Geometry: final body of the model. Coordinates: model frame, mm. A direction names the side the tool comes from. Coordinates: 2 decimals unless noted, no trailing zeros. Write each loop counter-clockwise with the first axis right and the second up, starting at its lowest first coordinate (ties: lowest second). Pieces come first, ordered by that corner, then holes. Notation, with made-up numbers: M 5,78.25 L 24,78.25 A27 cw 24,100.25 Z; hole C 19.5,25.25 d10. An arc over 180 degrees is marked long. Write item = value, one per line. Start each with the question number.
Item 1: Ray query, L1, parallel to Y at x = 10, z = -15.5; L2, parallel to Z at x = 24.75, y = -16.5; L3, parallel to Z at x = 15.5, y = -2. Return the intervals inside material, ascending. Write a range as [from, to].
Item 2: Section C-C on z = -13. Output: boundary loops of the cut face in (x, y), plus the area to 3 significant figures.
Item 3: Section A-A on x = 18.25. Output: boundary loops of the cut face in (y, z).
Item 4: First-contact query: pin 1 Ø10 at (x, y) = (11, -11.5) entering from +Z; pin 2 Ø5 at (x, y) = (13, 9.5) entering from +Z; pin 3 Ø4 at (x, y) = (16.5, 10.5) entering from +Z. Flat tips, straight axial feed; report the tip coordinate or a pass-through.
Item 5: Section B-B on y = 34. Output: boundary loops of the cut face in (x, z), plus the area to 3 significant figures.
Item 6: Reachability of faces 1 (the flat face through (13, -44.45, -20)), 2 (the flat face through (12.52, -41.77, -15.41)) from +Z, -Z, +X, -X, +Y, -Y: full face, straight path, thin tool, end or side. Return the list, or none.
from build123d import *

# Parameters (mm, degrees)
F1_DEPTH = 25.4
F2_R     = 5.08


with BuildPart() as f1:
    # F0 (on Right) → F1 (new body)
    with BuildSketch(Plane.YZ):
        Polygon((-44.45, -15.24), (-44.45, -25.4), (44.45, -25.4), (44.45, 22.65116), (24.805692, 13.670905), (-41.259935, -16.530525), (-42.299335, -14.256839), align=None)
    extrude(amount=F1_DEPTH)

    # F2
    f2_edges = [f1.edges().sort_by_distance(p)[0] for p in [
        (12.7, 44.45, 22.65116),
    ]]
    fillet(f2_edges, radius=F2_R)


solid = f1.part
Responses:
q1.L1 = [-44.45, -41.73], [-39.01, 44.45]
q1.L2 = [-25.4, -5.21]
q1.L3 = [-25.4, 1.42]
q2.outline = M 0,-33.54 L 25.4,-33.54 L 25.4,44.45 L 0,44.45 Z
q2.area = 1,980 mm²
q3.outline = M -44.45,-25.4 L 44.45,-25.4 L 44.45,14.74 A5.08 ccw 37.26,19.36 L -41.26,-16.53 L -42.3,-14.26 L -44.45,-15.24 Z
q4.pin_1 = -0.64
q4.pin_2 = 7.82
q4.pin_3 = 8.05
q5.outline = M 0,-25.4 L 25.4,-25.4 L 25.4,17.87 L 0,17.87 Z
q5.area = 1,100 mm²
q6.face_1 = +Z, -Z, +X, -X, -Y
q6.face_2 = +Z, +X, -X
